Autodesk Inventor part; units mm, degrees
ref_plane "YZ Plane" through (0, 0, 0) normal (1, 0, 0) x (0, 1, 0)
ref_plane "XZ Plane" through (0, 0, 0) normal (0, 1, 0) x (-1, 0, 0)
ref_plane "XY Plane" through (0, 0, 0) normal (0, 0, 1) x (1, 0, 0)
sketch "Sketch1" plane through (0, 0, 0) normal (0, 0, 1) x (1, 0, 0)
  line L0 (-50, -25) -> (50, -25)
  line L1 (50, -25) -> (50, 25)
  line L2 (50, 25) -> (-50, 25)
  line L3 (-50, 25) -> (-50, -25)
  line L4 (-50, -25) -> (50, 25) construction
  line L5 (50, -25) -> (-50, 25) construction
  circle A0 centre (44, 19) radius 1.6
  line L6 (0, 35.5799) -> (0, -35.5799)
  line L7 (-70.5799, 0) -> (70.5799, 0)
  circle A1 centre (44, 19) radius 5 construction
  circle A2 centre (-44, 19) radius 1.6
  circle A3 centre (-44, 19) radius 5 construction
  circle A4 centre (44, -19) radius 1.6
  circle A5 centre (44, -19) radius 5 construction
  circle A6 centre (-44, -19) radius 1.6
  circle A7 centre (-44, -19) radius 5 construction
  circle A8 centre (40, 0) radius 10
  line L8 (40, 10) -> (50, 10)
  line L9 (40, -10) -> (50, -10)
  point P0 (0, 0)
  dimension "d0" = 100
  dimension "d1" = 50
  dimension "d2" = 6
  dimension "d3" = 6
  dimension "d4" = 3.2
  dimension "d5" = 10
  dimension "d9" = 20
  dimension "d10" = 10
extrude "Extrusion1" add sketch "Sketch1" along normal blind 1.6 contours L3 L7 L6 L0 | L6 L7 A8 L9 L1 L0 | L3 L2 L6 L7 | L6 L2 L1 L8 A8 L7
fillet "Fillet1" radius 2 4 edges at (-50, 25, 0.8) (50, 25, 0.8) (50, -25, 0.8) (-50, -25, 0.8)
sketch "MCU_Power_PCB_Outline" plane through (0, 0, 1.6) normal (0, 0, 1) x (1, 0, 0)
  arc A0 (-50, -23) -> (-48, -25) centre (-48, -23) ccw
  line L0 (-48, -25) -> (48, -25)
  arc A1 (48, -25) -> (50, -23) centre (48, -23) ccw
  line L1 (50, -23) -> (50, -10)
  arc A2 (50, 23) -> (48, 25) centre (48, 23) ccw
  line L2 (48, 25) -> (-48, 25)
  arc A3 (-48, 25) -> (-50, 23) centre (-48, 23) ccw
  line L3 (-50, 23) -> (-50, -23)
  circle A4 centre (-44, -19) radius 1.6
  circle A5 centre (44, -19) radius 1.6
  circle A6 centre (44, 19) radius 1.6
  circle A7 centre (-44, 19) radius 1.6
  line L4 (50, -10) -> (40, -10)
  arc A8 (40, 10) -> (40, -10) centre (40, 0) ccw
  line L5 (40, 10) -> (50, 10)
  line L6 (50, 10) -> (50, 23)
  point P0 (0, 0)
equation "\"d3\" = d2"
properties part number "MCU_Power_PCB"
Design review of the part built by this model. Coordinates are the model's own, in mm. Give positions to 0.01 mm unless a question says otherwise; leave off trailing zeros. Write each loop counter-clockwise with the first axis right and the second up, starting at its lowest first coordinate (ties: lowest second). Pieces come first, ordered by that corner, then holes. Notation, with made-up numbers: M -18.5,-29.5 L 40.5,-29.5 A14 ccw 40.5,-18.5 Z; hole C 14,65.25 d9. An arc over 180 degrees is marked long. Return JSON: item names as keys, results as strings. Group by question number.
Item 1: Take a section at B-B (z = 0.4). Give the boundary of the cut face in (x, y), plus the area to 3 significant figures.
Item 2: Take a section at A-A (x = -44). Give the boundary of the cut face in (y, z), plus the area to 3 significant figures.
Item 3: Take a section at C-C (y = 19). Give the boundary of the cut face in (x, z).
Item 4: Clearance check with a flat-ended pin moving along its axis: pin 1 Ø4 at (x, y) = (44, -19) entering from -Z. State where the tip first meets the part, or that it passes through.
Item 5: Wall thickness on line 1 along Y through (x, z) = (44, 1.05); line 2 along Y through (x, z) = (-44, 1.1); line 3 along Y through (x, z) = (45, 1.15): over which ranges is each line inside the solid? List them lowest first.
Item 6: Take a section at D-D (x = 44). Give the boundary of the cut face in (y, z), plus the area to 3 significant figures.
Item 7: The part is to be moulded in two halves that separate along X. For faces 1 (the flat face through (-1, 0, 0)), 2 (the cylindrical face through (30, 0, 1)), 3 (the cylindrical face through (43.792, 17.414, 0.789)), 4 (the cylindrical face through (-49.4, 24.43, 0.81)), say which applies: pulls with the +X half, pulls with the -X half, needs draft (parallel to the pull), parting line crosses it, or undercut.
Return value:
{
 "1": {"outline": "M -50,-23 A2 ccw -48,-25 L 48,-25 A2 ccw 50,-23 L 50,-10 L 40,-10 A10 cw 40,10 L 50,10 L 50,23 A2 ccw 48,25 L -48,25 A2 ccw -50,23 Z; hole C -44,-19 d3.2; hole C -44,19 d3.2; hole C 44,-19 d3.2; hole C 44,19 d3.2", "area": "4,610 mm2"},
 "2": {"outline": "M -25,0 L -20.6,0 L -20.6,1.6 L -25,1.6 Z; M -17.4,0 L 17.4,0 L 17.4,1.6 L -17.4,1.6 Z; M 20.6,0 L 25,0 L 25,1.6 L 20.6,1.6 Z", "area": "69.8 mm2"},
 "3": {"outline": "M -50,0 L -45.6,0 L -45.6,1.6 L -50,1.6 Z; M -42.4,0 L 42.4,0 L 42.4,1.6 L -42.4,1.6 Z; M 45.6,0 L 50,0 L 50,1.6 L 45.6,1.6 Z"},
 "4": {"pin 1": "stops at z = 0"},
 "5": {"line 1": "y = -25 to -20.6, -17.4 to -10, 10 to 17.4, 20.6 to 25", "line 2": "y = -25 to -20.6, -17.4 to 17.4, 20.6 to 25", "line 3": "y = -25 to -20.25, -17.75 to -10, 10 to 17.75, 20.25 to 25"},
 "6": {"outline": "M -25,0 L -20.6,0 L -20.6,1.6 L -25,1.6 Z; M -17.4,0 L -10,0 L -10,1.6 L -17.4,1.6 Z; M 10,0 L 17.4,0 L 17.4,1.6 L 10,1.6 Z; M 20.6,0 L 25,0 L 25,1.6 L 20.6,1.6 Z", "area": "37.8 mm2"},
 "7": {"face 1": "needs draft", "face 2": "pulls with the +X half", "face 3": "undercut", "face 4": "pulls with the -X half"}
}
